from build123d import *

# Parameters (mm, degrees)
F1_DEPTH = 134.62
F2_DEPTH = 89.154
F3_R     = 7.871318
F5_DEPTH = 98.0821
F4_R     = 7.580211
F6_DEPTH = 98.0821


with BuildPart() as f1:
    # F0 (on Front) → F1 (new body, symmetric)
    with BuildSketch(Plane.XZ):
        with BuildLine():
            Line((-21.845277, 49.040429), (-37.894871, 49.040429))
            ThreePointArc((-37.894871, 49.040429), (0, 11.145558), (37.894871, 49.040429))
            Line((37.894871, 49.040429), (21.845277, 49.040429))
            ThreePointArc((21.845277, 49.040429), (0, 27.195152), (-21.845277, 49.040429))
        make_face()
    extrude(amount=F1_DEPTH, both=True)

    # F0 (on Front) → F2 (join, symmetric)
    with BuildSketch(Plane.XZ):
        with BuildLine():
            Line((-37.894871, 49.040429), (-61.969265, 49.040429))
            Line((-61.969265, 49.040429), (-61.969265, -49.040429))
            Line((-61.969265, -49.040429), (61.969265, -49.040429))
            Line((61.969265, -49.040429), (61.969265, 49.040429))
            Line((61.969265, 49.040429), (37.894871, 49.040429))
            ThreePointArc((37.894871, 49.040429), (0, 11.145558), (-37.894871, 49.040429))
        make_face()
    extrude(amount=F2_DEPTH, both=True)

    # F3 (on face) → F5 (cut)
    with BuildSketch(Plane.XY.offset(49.040429)):
        with Locations((-49.932068, 0)):
            Circle(F3_R)
    extrude(amount=-F5_DEPTH, mode=Mode.SUBTRACT)

    # F4 (on face) → F6 (cut)
    with BuildSketch(Plane.XY.offset(49.040429)):
        with Locations((49.932068, 0)):
            Circle(F4_R)
    extrude(amount=-F6_DEPTH, mode=Mode.SUBTRACT)


solid = f1.part
Source: CAD feature listing. Evaluate the final solid. Frame: model axes, mm. A direction names the side the tool comes from. Round coordinates to 2 decimals unless told otherwise and drop trailing zeros. Loops run counter-clockwise (first coordinate to the right, second up) from the corner with the lowest first, then second, coordinate; pieces in that order, holes last. Notation, with made-up numbers: (69.25, 65) - (93.25, 65) arc R19 ccw to (93.25, 91) - close; hole circle Ø11 at (4, 87). An arc over 180 degrees is marked (long way). Write item = value, one per line. Start each with the question number.
(1) Set-up query: faces 5 (the face through (-0.833, 111.569, 11.155)), 6 (the face through (-1, -1, -49.04)). Return all of +Z, -Z, +X, -X, +Y, -Y with unobstructed straight access to the full face (end or side cutting, diameter ignored); none if empty.
(2) Section query B-B, the plane z = 33. Output: boundary loops of the cut face in (x, y), plus the area to 3 significant figures.
(3) Pull-direction query (X, two-part tool) for faces 1 (the face through (-1, -89.154, -10)), 2 (the face through (-0.833, -112.205, 11.155)), 3 (the face through (42.36, 0.33, 0.69)), 4 (the face through (-57.796, 0.346, 0.687)); classes: +X half, -X half, draft (parallel to the pull), parting line (faces both ways), or undercut.
(4) Section query D-D, the plane y = -43. Output: boundary loops of the cut face in (x, z).
(5) Pin query (flat end, axial travel): pin 1 (4 mm diameter, centred on x = -6.5, y = 98.5, fed in from -Z); pin 2 (6 mm diameter, centred on x = 37.5, z = -12, fed in from -Y); pin 3 (10 mm diameter, centred on x = 3, z = -29, fed in from +Y). Return the tip coordinate at first contact, or that it passes through.
(6) Section query A-A, the plane y = 0. Output: boundary loops of the cut face in (x, z), plus the area to 3 significant figures.
(7) Ray query, line 1 along X through (y, z) = (85, 41); line 2 along Y through (x, z) = (34.5, -31); line 3 along Y through (x, z) = (-54.5, -2). Return the intervals inside material, ascending. Write a range as from..to.
(8) Section query C-C, the plane x = 48.5. Output: boundary loops of the cut face in (y, z).
Conclusion:
q1.face_5 = -Z, +Y
q1.face_6 = -Z, +X, -X, +Y, -Y
q2.outline = (-61.97, -89.15) - (-34.33, -89.15) - (-34.33, -134.62) - (-14.83, -134.62) - (-14.83, 134.62) - (-34.33, 134.62) - (-34.33, 89.15) - (-61.97, 89.15) - close; (14.83, -134.62) - (34.33, -134.62) - (34.33, -89.15) - (61.97, -89.15) - (61.97, 89.15) - (34.33, 89.15) - (34.33, 134.62) - (14.83, 134.62) - close; hole circle Ø15.74 at (-49.93, 0); hole circle Ø15.16 at (49.93, 0)
q2.area = 20,000 mm2
q3.face_1 = draft
q3.face_2 = parting line
q3.face_3 = undercut
q3.face_4 = undercut
q4.outline = (-61.97, -49.04) - (61.97, -49.04) - (61.97, 49.04) - (21.85, 49.04) arc R21.85 cw to (-21.85, 49.04) - (-61.97, 49.04) - close
q5.pin_1 = 11.41
q5.pin_2 = -89.15
q5.pin_3 = 89.15
q6.outline = (-61.97, -49.04) - (-57.8, -49.04) - (-57.8, 49.04) - (-61.97, 49.04) - close; (-42.06, -49.04) - (42.35, -49.04) - (42.35, 49.04) - (21.85, 49.04) arc R21.85 cw to (-21.85, 49.04) - (-42.06, 49.04) - close; (57.51, -49.04) - (61.97, -49.04) - (61.97, 49.04) - (57.51, 49.04) - close
q6.area = 8,380 mm2
q7.line_1 = -61.97..-20.31, 20.31..61.97
q7.line_2 = -89.15..89.15
q7.line_3 = -89.15..-6.41, 6.41..89.15
q8.outline = (-89.15, -49.04) - (-7.44, -49.04) - (-7.44, 49.04) - (-89.15, 49.04) - close; (7.44, -49.04) - (89.15, -49.04) - (89.15, 49.04) - (7.44, 49.04) - close
